Design review of the part built by this model. Coordinates are the model's own, in mm. Face numbers are marked on the shaded views. A direction names the side the tool comes from. Round coordinates to 2 decimals unless told otherwise and drop trailing zeros. Loops run counter-clockwise (first coordinate to the right, second up) from the corner with the lowest first, then second, coordinate; pieces in that order, holes last. Notation, with made-up numbers: (45.5, 37.25) - (78.5, 37.25) arc R10 cw to (78.5, 52.25) - close; hole circle Ø9 at (-33.75, 25). An arc over 180 degrees is marked (long way). Answer as CSV lines item,"result". Start each with the question number.
(1) Mouldability with a two-part tool opening along X and no side actions: class the marked faces 1, 2 and 3 as released by +X, released by -X, zero draft, split by the parting line, or undercut.
(2) Consider section A-A (z = 64). Give the boundary of the cut face in (x, y).
(3) Consider section C-C (x = 22). Give the boundary of the cut face in (y, z), and give its area (3 significant figures).
(4) Consider section B-B (y = -12.5). Give the boundary of the cut face in (x, z).
(5) For P1, Ø23, axis at x = -6.5, y = -7, coming from the +Z side, flat-tipped, find the tip position at first contact; note if it passes through.
(6) Wall thickness on L1, parallel to X at y = -24, z = 18; L2, parallel to Z at x = 31.5, y = -33: over which ranges is each line inside the solid? List them lowest first.
(7) For the marked faces 4 and 5, list the 3-axis set-ups (+Z, -Z, +X, -X, +Y, -Y) from which the entire face can be reached by the end or side of a thin tool; tool diameter is ignored.
Autodesk Fusion 360 part; units mm, degrees
sketch "Sketch1" plane through (0, 0, 0) normal (0, 0, 1) x (1, 0, 0)
  line L0 (38.1, 38.1) -> (-38.1, 38.1)
  line L1 (-38.1, 38.1) -> (-38.1, -38.1)
  line L2 (-38.1, -38.1) -> (38.1, -38.1)
  line L3 (38.1, -38.1) -> (38.1, 38.1)
  line L4 (38.1, 38.1) -> (-38.1, -38.1) construction
  line L5 (-38.1, 38.1) -> (38.1, -38.1) construction
  line L6 (-38.1, 38.1) -> (-45.72, 38.1)
  line L7 (-45.72, 38.1) -> (-45.72, -38.1)
  line L8 (-45.72, -38.1) -> (-38.1, -38.1)
  line L9 (-38.1, -38.1) -> (-38.1, 38.1)
  line L10 (38.1, 38.1) -> (45.72, 38.1)
  line L11 (45.72, 38.1) -> (45.72, -38.1)
  line L12 (45.72, -38.1) -> (38.1, -38.1)
  line L13 (38.1, -38.1) -> (38.1, 38.1)
  dimension "d1" = 76.2
  dimension "d2" = 76.2
  dimension "d3" = 7.62
extrude "Extrude1" add sketch "Sketch1" along normal blind 6.35 contours L0 L1 L2 L3 L9 L13
sketch "Sketch2" plane through (0, 0, 0) normal (0, 0, 1) x (1, 0, 0)
extrude "Extrude2" add sketch "Sketch1" along normal blind 76.2 contours L3 L10 L11 L12 L13 | L1 L6 L7 L8 L9
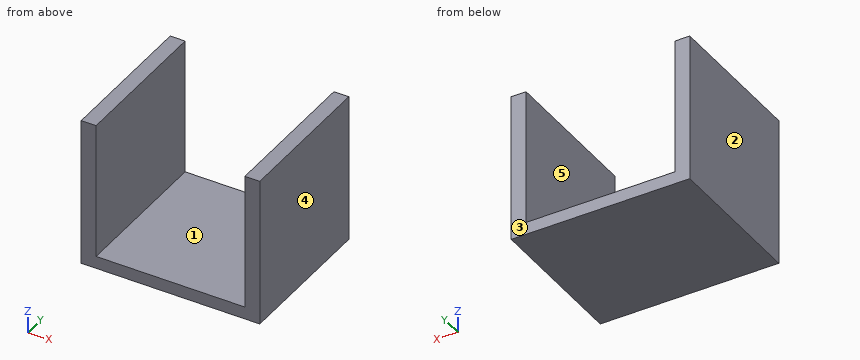
Determined:
1,face 1,"undercut"
1,face 2,"released by -X"
1,face 3,"zero draft"
2,outline,"(-45.72, -38.1) - (-38.1, -38.1) - (-38.1, 38.1) - (-45.72, 38.1) - close; (38.1, -38.1) - (45.72, -38.1) - (45.72, 38.1) - (38.1, 38.1) - close"
3,outline,"(-38.1, 0) - (38.1, 0) - (38.1, 6.35) - (-38.1, 6.35) - close"
3,area,"484 mm^2"
4,outline,"(-45.72, 0) - (45.72, 0) - (45.72, 76.2) - (38.1, 76.2) - (38.1, 6.35) - (-38.1, 6.35) - (-38.1, 76.2) - (-45.72, 76.2) - close"
5,P1,"stops at z = 6.35"
6,L1,"x = -45.72 to -38.1, 38.1 to 45.72"
6,L2,"z = 0 to 6.35"
7,face 4,"+Z, -Z, +X, +Y, -Y"
7,face 5,"+Z, +Y, -Y"
